Autodesk Inventor part; units mm, degrees
ref_plane "断面平面" through (-18.901655, -2.735635, 0) normal (0.1432375, -0.9896883, 0) x (0, 0, 1)
ref_plane "作業平面2" through (0, 0, 0) normal (-1, 0, 0) x (0, 0, 1)
ref_plane "作業平面3" through (8.401537, -124.717337, 0) normal (-0.4316004, 0.9020649, 0) x (0, 0, 1)
sketch "スケッチ パス" plane through (0, 0, 0) normal (0, 0, 1) x (1, 0, 0)
  arc A0 (19.09858, 0.022721) -> (-18.901655, -2.735635) centre (0, 0) ccw
  arc A1 (18.716428, -76.913324) -> (19.18706, -74.351396) centre (12.025093, -74.359916) ccw
  arc A2 (8.519671, -103.634445) -> (8.887698, -107.441661) centre (12.537104, -105.167493) ccw
  arc A3 (-1.049291, -126.085154) -> (16.506016, -119.666943) centre (8.401537, -124.717337) ccw
  line L0 (-1.049291, -126.085154) -> (-18.901655, -2.735635)
  line L1 (19.09858, 0.022721) -> (19.18706, -74.351396)
  line L2 (18.716428, -76.913324) -> (8.519671, -103.634445)
  line L3 (8.887698, -107.441661) -> (16.506016, -119.666943)
ref_plane "断面平面" through (-18.901655, -2.735635, 0) normal (0.1432375, -0.9896883, 0) x (0, 0, 1)
ref_plane "作業平面2" through (0, 0, 0) normal (-1, 0, 0) x (0, 0, 1)
ref_plane "作業平面3" through (8.401537, -124.717337, 0) normal (-0.4316004, 0.9020649, 0) x (0, 0, 1)
ref_plane "作業平面4" through (12.025093, -74.359916, 0) normal (0.0892463, 0.9960096, 0) x (0, 0, 1)
sketch "断面" plane through (-18.901655, -2.735635, 0) normal (0.1432375, -0.9896883, 0) x (0, 0, 1)
  line L0 (-4, 0.3) -> (4, 0.3)
  line L1 (4, 0.3) -> (4, -0.3)
  line L2 (4, -0.3) -> (-4, -0.3)
  line L3 (-4, -0.3) -> (-4, 0.3)
  line L4 (-4, 0) -> (4, 0) construction
  point P0 (0, 0)
  point P1 (0, 0)
  dimension "d0" = 8
  dimension "d4" = 0.3
  dimension "d5" = 0.3
sweep "ベルト" add profiles "断面" path "スケッチ パス"
equation "\"d4\" = da_a"
equation "\"d5\" = da_a2"
equation "\"da_B\" = 6"
equation "\"da_pb\" = 2.5"
equation "\"da_L\" = 345.26878"
equation "\"da_a\" = 0.3"
equation "\"da_S\" = 1.5"
equation "\"da_Beta\" = 20deg"
equation "\"da_Ht\" = 0.7"
equation "\"da_H\" = 1.3"
equation "\"da_a2\" = 0.3"
properties part number "歯付きベルト" material "Rubber"
Here's how the part is built. I have some questions about the finished solid (model axes, mm). A direction names the side the tool comes from. Round coordinates to 2 decimals unless told otherwise and drop trailing zeros. Loops run counter-clockwise (first coordinate to the right, second up) from the corner with the lowest first, then second, coordinate; pieces in that order, holes last.
1. If we section it at A-A on z = -0.25: Write out the boundary of the cut face in (x, y), plus the area to 3 significant figures.
Answer list:
outline: (-19.2, -2.78) - (-1.35, -126.13) arc R9.85 ccw (long way) to (16.76, -119.51) - (9.14, -107.28) arc R4 cw to (8.8, -103.74) - (19, -77.02) arc R7.46 ccw to (19.49, -74.35) - (19.4, 0.02) arc R19.4 ccw (long way) to start; hole (-18.6, -2.69) - (-0.75, -126.04) arc R9.25 ccw (long way) to (16.25, -119.83) - (8.63, -107.6) arc R4.6 cw to (8.24, -103.53) - (18.44, -76.81) arc R6.86 ccw to (18.89, -74.35) - (18.8, 0.02) arc R18.8 ccw (long way) to start
area: 207 mm2
2. Which directions (+Z, -Z, +X, -X, +Y, -Y) give clear straight access to the entire face, cutting with the end or side of a thin tool? Please do faces 1 (the face through (-12.8, -45.8, -4)), 2 (the face through (-0.93, 18.776, 0.056)), 3 (the face through (12.9, -113.31, 0.06)).
Answer list:
face 1: -Z, +X, -X, +Y, -Y
face 2: +Z, -Z
face 3: +Z, -Z, +X
3. If I drill on line 1 along X through (y, z) = (-115.5, 1.25); line 2 along X through (y, z) = (-53, -2); line 3 along Y through (x, z) = (3.5, 1.5), over which ranges is the centre line in solid material (lowest first)?
Answer list:
line 1: x = -2.88 to -2.28, 13.56 to 14.26
line 2: x = -11.93 to -11.32, 18.86 to 19.46
line 3: y = -133.26 to -132.56, 18.47 to 19.08
4. We'd pull the mould along Y, two halves only. Please class faces 4 (the face through (-10.1, -62.9, 4)), 5 (the face through (-9.554, -65.231, -0.056)), 6 (the face through (-10.147, -65.317, 0.056)): +Y half, -Y half, draft (parallel to the pull), parting line (faces both ways), or undercut.
Answer list:
face 4: draft
face 5: undercut
face 6: -Y half
5. If we section it at B-B on y = -109.5: Write out the boundary of the cut face in (x, z), plus the area to 3 significant figures.
Answer list:
outline: (-3.75, -4) - (-3.15, -4) - (-3.15, 4) - (-3.75, 4) - close; (9.82, -4) - (10.52, -4) - (10.52, 4) - (9.82, 4) - close
area: 10.5 mm2
6. For P1, Ø1.5, axis at y = -86.5, z = -2, coming from the -X side; P2, Ø1.5, axis at x = -14, z = -2, coming from the +Y side; P3, Ø4, axis at y = -30.5, z = -3, coming from the -X side, each with a flat end and sliding along its axis, tell me the tip position at first contact or that it passes through.
Answer list:
P1: stops at x = -7.19
P2: stops at y = 14.17
P3: stops at x = -15.48
7. If we section it at C-C on x = -6.5: Write out the boundary of the cut face in (y, z).
Answer list:
outline: (-90.52, -4) - (-86.33, -4) - (-86.33, 4) - (-90.52, 4) - close; (17.64, -4) - (18.28, -4) - (18.28, 4) - (17.64, 4) - close
